Source: CAD feature listing. Evaluate the final solid. Frame: model axes, mm. A direction names the side the tool comes from. Round coordinates to 2 decimals unless told otherwise and drop trailing zeros. Write each loop counter-clockwise with the first axis right and the second up, starting at its lowest first coordinate (ties: lowest second). Pieces come first, ordered by that corner, then holes. Notation, with made-up numbers: M -5.75,26.25 L 4.25,26.25 A14 cw 4.25,51.25 Z; hole C 26,-37.5 d6. An arc over 180 degrees is marked long. Answer in a Markdown table with one row per item.
from build123d import *

# Parameters (mm, degrees)
SKETCH_1_R          = 30
EXTRUDE_1_DEPTH     = 8
SKETCH_2_R          = 2.5
CUT_EXTRUDE_1_DEPTH = 50
SKETCH_3_R          = 2.5
CUT_EXTRUDE_2_DEPTH = 20


with BuildPart() as part:
    # 草图1 → 凸台-拉伸1 (new body)
    with BuildSketch(Plane.XY):
        with BuildLine():
            Line((-48, 114), (-48, 0))
            Line((-48, 0), (48, 0))
            Line((48, 0), (48, 114))
            ThreePointArc((48, 114), (0, 150), (-48, 114))
        make_face()
        with Locations((0, 100)):
            Circle(SKETCH_1_R, mode=Mode.SUBTRACT)
    extrude(amount=EXTRUDE_1_DEPTH)

    # 草图2 → 切除-拉伸1 (cut)
    with BuildSketch(Plane.XZ):
        with Locations(Location((35, 4, 0), (0, 0, 270))):
            Circle(SKETCH_2_R)
        with Locations(Location((-35, 4, 0), (0, 0, 270))):
            Circle(SKETCH_2_R)
    extrude(amount=-CUT_EXTRUDE_1_DEPTH, mode=Mode.SUBTRACT)

    # 草图3 → 切除-拉伸2 (cut)
    with BuildSketch(Plane.XY.offset(8)):
        with Locations((0, 40)):
            Circle(SKETCH_3_R)
    extrude(amount=-CUT_EXTRUDE_2_DEPTH, mode=Mode.SUBTRACT)


solid = part.part
Q1. Section A-A (y = 40). Return loops of the section in (x, z).
Solutions:
| item | result |
|---|---|
| outline | M -48,0 L -2.5,0 L -2.5,8 L -48,8 Z; M 2.5,0 L 48,0 L 48,8 L 2.5,8 Z; hole C -35,4 d5; hole C 35,4 d5 |
Q2. Pull-direction query (X, two-part tool) for faces 3 (the flat face through (-48, 58, 4)), 4 (the cylindrical face through (-0.54, 37.56, 4.06)), 5 (the flat face through (-1, 59, 0)); classes: pulls with the +X half, pulls with the -X half, needs draft (parallel to the pull), parting line crosses it, or undercut.
Solutions:
| item | result |
|---|---|
| face 3 | pulls with the -X half |
| face 4 | undercut |
| face 5 | needs draft |
Q3. Contact query for flat-ended pins moving along their axis: pin 1 Ø2 at (x, z) = (-7, 6) entering from +Y; pin 2 Ø2.5 at (x, z) = (36, 3.5) entering from -Y; pin 3 Ø8 at (x, y) = (-15, 81.5) entering from -Z (1 decimal); pin 4 Ø4.5 at (x, z) = (-35, 4) entering from +Y. Output: stop coordinate, or through.
Solutions:
| item | result |
|---|---|
| pin 1 | stops at y = 149.64 |
| pin 2 | stops at y = 50 |
| pin 3 | passes through |
| pin 4 | stops at y = 137.78 |
Q4. Access query for faces 1 (the flat face through (-1, 0, 4)), 2 (the flat face through (-35, 50, 4)). Directions: +Z, -Z, +X, -X, +Y, -Y. A direction counts if a zero-diameter tool reaches every point of the face in a straight line with its end or side. Return the directions, or none.
Solutions:
| item | result |
|---|---|
| face 1 | +Z, -Z, +X, -X, -Y |
| face 2 | -Y |
Q5. Section B-B (z = 4). Return loops of the section in (x, y).
Solutions:
| item | result |
|---|---|
| outline | M -48,0 L -37.5,0 L -37.5,50 L -32.5,50 L -32.5,0 L 32.5,0 L 32.5,50 L 37.5,50 L 37.5,0 L 48,0 L 48,114 A50 ccw -48,114 Z; hole C 0,100 d60; hole C 0,40 d5 |
Q6. Material intervals for probe 1 along X at (y, z) = (34.5, 4); probe 2 along X at (y, z) = (10.5, 3.25); probe 3 along Y at (x, z) = (2, 7.25), sorted ascending.
Solutions:
| item | result |
|---|---|
| probe 1 | x = -48 to -37.5, -32.5 to 32.5, 37.5 to 48 |
| probe 2 | x = -48 to -37.38, -32.62 to 32.62, 37.38 to 48 |
| probe 3 | y = 0 to 38.5, 41.5 to 70.07, 129.93 to 149.96 |
Q7. Section C-C (x = 0). Return loops of the section in (y, z), and give its area (3 significant figures).
Solutions:
| item | result |
|---|---|
| outline | M 0,0 L 37.5,0 L 37.5,8 L 0,8 Z; M 42.5,0 L 70,0 L 70,8 L 42.5,8 Z; M 130,0 L 150,0 L 150,8 L 130,8 Z |
| area | 680 mm2 |
Q8. Section D-D (x = 28.5). Return loops of the section in (y, z).
Solutions:
| item | result |
|---|---|
| outline | M 0,0 L 90.63,0 L 90.63,8 L 0,8 Z; M 109.37,0 L 141.08,0 L 141.08,8 L 109.37,8 Z |
